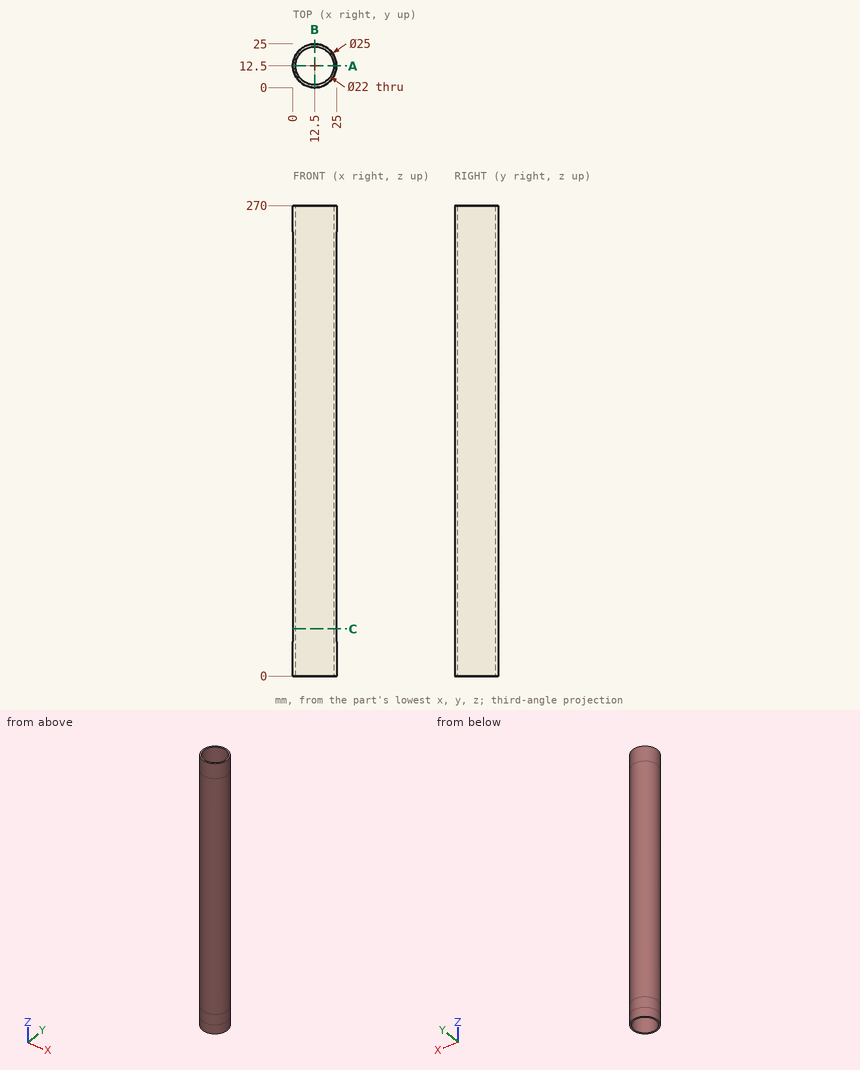
Input: dimensioned drawing with shaded views. Units: mm. Origin: part minimum x, y, z. Round coordinates to 2 decimals unless told otherwise and drop trailing zeros. Loops run counter-clockwise (first coordinate to the right, second up) from the corner with the lowest first, then second, coordinate; pieces in that order, holes last. Notation, with made-up numbers: (82, 0) -> (139, 0) arc R18 cw to (139, 33) -> close; hole circle Ø7 at (-35, -11). An arc over 180 degrees is marked (long way). Answer as a JSON object with one key per item and string values. Group by question number.
Q1. Section query C-C (z = 27). Output: boundary loops of the cut face in (x, y), plus the area to 3 significant figures.
Q2. Section query A-A (y = 12.5). Output: boundary loops of the cut face in (x, z), plus the area to 3 significant figures.
Q3. Ray query, line 1 (Y direction, x = 12.5, z = 124); line 2 (Y direction, x = 6.25, z = 71); line 3 (X direction, y = 20, z = 139). Return the intervals inside material, ascending. Write a range as from..to.
Q4. Contact query for flat-ended pins moving along their axis: P1, Ø12, axis at y = 4.5, z = 213.5, coming from the +X side; P2, Ø3, axis at x = 19.5, z = 64.5, coming from the -Y side (3 decimals); P3, Ø10, axis at x = 16, z = 95.5, coming from the +Y side; P4, Ø8, axis at x = 14.5, y = 6.5, coming from the +Z side. Output: stop coordinate, or through.
Completed:
{
 "1": {"outline": "circle Ø25 at (12.5, 12.5); hole circle Ø22 at (12.5, 12.5)", "area": "111 mm²"},
 "2": {"outline": "(0, 0) -> (1.5, 0) -> (1.5, 270) -> (0, 270) -> close; (23.5, 0) -> (25, 0) -> (25, 270) -> (23.5, 270) -> close", "area": "810 mm²"},
 "3": {"line 1": "0..1.5, 23.5..25", "line 2": "1.67..3.45, 21.55..23.33", "line 3": "2.5..4.45, 20.55..22.5"},
 "4": {"P1": "x = 24.84", "P2": "y = 1.275", "P3": "y = 25", "P4": "through"}
}
